from build123d import *

# Parameters (mm, degrees)
F0_W        = 88.9
F0_H        = 165.1
F1_DEPTH    = 6.35
F2_DEPTH    = 25.4
F3_DEPTH    = 50.8
F4_C1_SIZE2 = 7.3323484187
F4_C1_SIZE  = 12.7
F4_C2_SIZE2 = 12.7
F4_C2_SIZE  = 7.3323484187
F4_C3_SIZE2 = 12.7
F4_C3_SIZE  = 7.3323484187
F4_C4_SIZE2 = 7.3323484187
F4_C4_SIZE  = 12.7


with BuildPart() as f1:
    # F0 (on Top) → F1 (new body)
    with BuildSketch(Plane.XY):
        Rectangle(F0_W, F0_H)
        Polygon((38.1, 38.1), (38.1, -76.2), (0, -76.2), (-38.1, -76.2), (-38.1, -38.1), (-38.1, 76.2), (0, 76.2), (38.1, 76.2), align=None, mode=Mode.SUBTRACT)
    extrude(amount=F1_DEPTH)

    # F0 (on Top) → F2 (join)
    with BuildSketch(Plane.XY):
        with BuildLine():
            Line((0, -76.2), (38.1, -76.2))
            Line((38.1, -76.2), (38.1, 38.1))
            Line((38.1, 38.1), (12.7, 38.1))
            ThreePointArc((12.7, 38.1), (3.7197438789, 41.8197438789), (0, 50.8))
            Line((0, 50.8), (0, 76.2))
            Line((0, 76.2), (-38.1, 76.2))
            Line((-38.1, 76.2), (-38.1, -38.1))
            Line((-38.1, -38.1), (-12.7, -38.1))
            ThreePointArc((-12.7, -38.1), (-3.7197438789, -41.8197438789), (0, -50.8))
            Line((0, -50.8), (0, -76.2))
        make_face()
    extrude(amount=F2_DEPTH)

    # F0 (on Top) → F3 (join)
    with BuildSketch(Plane.XY):
        with BuildLine():
            Line((-38.1, -76.2), (0, -76.2))
            Line((0, -76.2), (0, -50.8))
            ThreePointArc((0, -50.8), (-3.7197438789, -41.8197438789), (-12.7, -38.1))
            Line((-12.7, -38.1), (-38.1, -38.1))
            Line((-38.1, -38.1), (-38.1, -76.2))
        make_face()
        with BuildLine():
            Line((12.7, 38.1), (38.1, 38.1))
            Line((38.1, 38.1), (38.1, 76.2))
            Line((38.1, 76.2), (0, 76.2))
            Line((0, 76.2), (0, 50.8))
            ThreePointArc((0, 50.8), (3.7197438789, 41.8197438789), (12.7, 38.1))
        make_face()
    extrude(amount=F3_DEPTH)

    # F4: chamfer of 12.7 x 7.3323484187 on 4 edges, made by hand

    # F4_c1
    f4_c1_edges = [f1.edges().sort_by_distance(p)[0] for p in [
        (19.05, 76.2, 50.8),
    ]]
    f4_c1_side = f1.faces().sort_by_distance((19.05, 76.2, 50.6533530316))[0]
    chamfer(f4_c1_edges, length=F4_C1_SIZE, length2=F4_C1_SIZE2, reference=f4_c1_side)

    # F4_c2
    f4_c2_edges = [f1.edges().sort_by_distance(p)[0] for p in [
        (-19.05, -76.2, 50.8),
    ]]
    f4_c2_side = f1.faces().sort_by_distance((-19.05, -76.2, 50.6533530316))[0]
    chamfer(f4_c2_edges, length=F4_C2_SIZE, length2=F4_C2_SIZE2, reference=f4_c2_side)

    # F4_c3
    f4_c3_edges = [f1.edges().sort_by_distance(p)[0] for p in [
        (-38.1, -50.8, 50.8),
    ]]
    f4_c3_side = f1.faces().sort_by_distance((-38.1, -50.8, 50.6533530316))[0]
    chamfer(f4_c3_edges, length=F4_C3_SIZE, length2=F4_C3_SIZE2, reference=f4_c3_side)

    # F4_c4
    f4_c4_edges = [f1.edges().sort_by_distance(p)[0] for p in [
        (38.1, 53.4838257906, 50.8),
    ]]
    f4_c4_side = f1.faces().sort_by_distance((38.1, 53.4838257906, 50.6533530316))[0]
    chamfer(f4_c4_edges, length=F4_C4_SIZE, length2=F4_C4_SIZE2, reference=f4_c4_side)


solid = f1.part
Can you work these out from the model? Positions are in its coordinate system, mm. A direction names the side the tool comes from. Give positions to 0.01 mm unless a question says otherwise; leave off trailing zeros. Order: outer loops, then holes, each group sorted by start corner. A loop starts at its lowest first (then second) coordinate and runs counter-clockwise, first axis right, second up. Notation, with made-up numbers: M -9.5,7 L 22.5,7 A21 ccw 22.5,41 Z; hole C -12.5,25.25 d11. An arc over 180 degrees is marked long. Use one line per item in the form item = value. Start each with the question number.
Item 1: If I drill on line 1 along Y through (x, z) = (-31, 14); line 2 along X through (y, z) = (-52, 32); line 3 along Z through (x, y) = (10, -29.5), over which ranges is the centre line in solid material (lowest first)?
Item 2: If we section it at D-D (z = 46): Write out the boundary of the cut face in (x, y).
Item 3: If we section it at B-B (x = 17.5): Write out the boundary of the cut face in (y, z), then the cut area to 3 significant figures.
Item 4: If we section it at A-A (z = 28): Write out the boundary of the cut face in (x, y).
Item 5: Will these pins go through, and if not, where does the flat tip stop? pin 1 Ø20.5 at (x, z) = (-19.5, 41.5) entering from +Y; pin 2 Ø1.5 at (x, z) = (19, 23) entering from +Y; pin 3 Ø1 at (x, y) = (-29.5, 50) entering from +Z; pin 4 Ø8 at (x, y) = (15, -16.5) entering from -Z.
Item 6: If we section it at C-C (y = -5): Write out the boundary of the cut face in (x, z), then the cut area to 3 significant figures.
Item 7: For faces 1 (the flat face through (0, -64, 38)), 2 (the flat face through (-25, -38.1, 38)), 3 (the flat face through (-1, 1, 25.4)), which set-ups out of +Z, -Z, +X, -X, +Y, -Y let a thin tool reach every point of the face, with its end or its side?
Outcome:
q1.line_1 = -76.2 to 76.2
q1.line_2 = -38.1 to 0
q1.line_3 = 0 to 25.4
q2.outline = M -33.71,-71.81 L 0,-71.81 L 0,-50.8 A12.7 ccw -12.7,-38.1 L -33.71,-38.1 Z; M 0,50.8 A12.7 ccw 12.7,38.1 L 33.54,38.1 L 33.54,71.64 L 0,71.64 Z
q3.outline = M -82.55,0 L 82.55,0 L 82.55,6.35 L 76.2,6.35 L 76.2,38.1 L 68.87,50.8 L 38.1,50.8 L 38.1,25.4 L -76.2,25.4 L -76.2,6.35 L -82.55,6.35 Z
q3.area = 4,870 mm2
q4.outline = M -38.1,-76.2 L 0,-76.2 L 0,-50.8 A12.7 ccw -12.7,-38.1 L -38.1,-38.1 Z; M 0,50.8 A12.7 ccw 12.7,38.1 L 38.1,38.1 L 38.1,76.2 L 0,76.2 Z
q5.pin_1 = -38.1
q5.pin_2 = 76.2
q5.pin_3 = 25.4
q5.pin_4 = 0
q6.outline = M -44.45,0 L 44.45,0 L 44.45,6.35 L 38.1,6.35 L 38.1,25.4 L -38.1,25.4 L -38.1,6.35 L -44.45,6.35 Z
q6.area = 2,020 mm2
q7.face_1 = +Z, +X, -Y
q7.face_2 = +Z, +X, -X, +Y
q7.face_3 = +Z
